Part model, mm, in its own coordinate system. Face numbers are marked on the shaded views. A direction names the side the tool comes from. Coordinates: 2 decimals unless noted, no trailing zeros. Loops run counter-clockwise (first coordinate to the right, second up) from the corner with the lowest first, then second, coordinate; pieces in that order, holes last. Notation, with made-up numbers: M -14.75,68 L -10.75,68 A30 cw -10.75,101 Z; hole C 18.5,-13.5 d5. An arc over 180 degrees is marked long. Use a Markdown table: item, result. Add a question column.
1) Band-saw the part on A-A (z = 10.5). List the corners of the cut face in (x, y).
2) Wall check: probe 1 along X at (y, z) = (-4.5, 17.5); probe 2 along Z at (x, y) = (40, -8.25); probe 3 along X at (y, z) = (-2.25, 3). Give the ranges that are in metal, low to high. Write a range as from..to.
3) Pin check, flat tips, straight feed: pin 1 Ø2 at (x, y) = (33.5, -6.5) entering from +Z; pin 2 Ø1 at (y, z) = (-10, 11.5) entering from -X. Stop position of each tip, or through.
4) Band-saw the part on C-C (z = 18.75). List the corners of the cut face in (x, y), plus the area to 3 significant figures.
5) Pull direction Z, two halves, no side cores. Call the marked faces 3, 4 and 5: released by +Z, released by -Z, zero draft, split by the parting line, or undercut.
6) Tool access for the marked faces 1 and 2: list every direction of +Z, -Z, +X, -X, +Y, -Y with a clear straight run to the whole face (end or side of a thin tool).
7) Band-saw the part on D-D (x = 33.5). List the corners of the cut face in (y, z), plus the area to 3 significant figures.
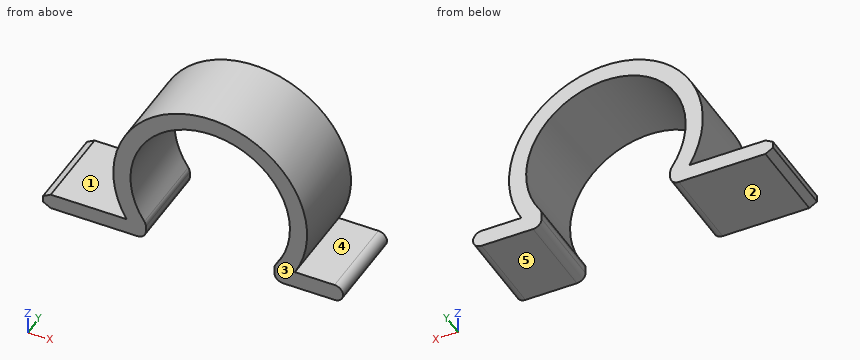
from build123d import *

# Parameters (mm, degrees)
F1_DEPTH   = 12.7
F2_SIZE2   = 0.6599113577
F2_SIZE    = 1.143
F2_2_SIZE2 = 0.6599113577
F2_2_SIZE  = 1.143
F3_R       = 1.26999


# Not quite as in the source:
# - a fillet or chamfer is up to 0.001 mm smaller than in the source, because OpenCascade refuses the exact size


with BuildPart() as f1:
    # F0 (on Front) → F1 (new body)
    with BuildSketch(Plane.XZ):
        with BuildLine():
            Line((0, 2.286), (0, 0))
            Line((0, 0), (15.24, 0))
            Line((15.24, 0), (15.24, 2.54))
            ThreePointArc((15.24, 2.54), (24.765, 21.336682776), (34.29, 2.54))
            Line((34.29, 2.54), (34.29, 0))
            Line((34.29, 0), (44.45, 0))
            Line((44.45, 0), (44.45, 2.54))
            Line((44.45, 2.54), (37.3021676826, 2.54))
            ThreePointArc((37.3021676826, 2.54), (24.6187816105, 23.8759379026), (12.3727573659, 2.286))
            Line((12.3727573659, 2.286), (0, 2.286))
        make_face()
    extrude(amount=F1_DEPTH)

    # F2
    f2_edges = [f1.edges().sort_by_distance(p)[0] for p in [
        (0, -6.35, 0),
    ]]
    f2_side = f1.faces().sort_by_distance((7.62, -6.35, 0))[0]
    chamfer(f2_edges, length=F2_SIZE, length2=F2_SIZE2, reference=f2_side)

    # F2#2
    f2_2_edges = [f1.edges().sort_by_distance(p)[0] for p in [
        (0, -6.35, 2.286),
    ]]
    f2_2_side = f1.faces().sort_by_distance((6.186379, -6.35, 2.286))[0]
    chamfer(f2_2_edges, length=F2_2_SIZE, length2=F2_2_SIZE2, reference=f2_2_side)

    # F3 (radius 1.27 in the source; OpenCascade refuses exactly that, so slightly less here)
    f3_edges = [f1.edges().sort_by_distance(p)[0] for p in [
        (44.45, -6.35, 2.54),
        (44.45, -6.35, 0),
        (34.29, -6.35, 0),
        (34.29, -6.35, 2.54),
        (15.24, -6.35, 2.54),
        (15.24, -6.35, 0),
    ]]
    fillet(f3_edges, radius=F3_R)


solid = f1.part
Entries:
| question | item | result |
|---|---|---|
| 1 | outline | M 10.45,-12.7 L 12.99,-12.7 L 12.99,0 L 10.45,0 Z; M 36.54,-12.7 L 39.08,-12.7 L 39.08,0 L 36.54,0 Z |
| 2 | probe 1 | 12.83..16.05, 33.48..36.7 |
| 2 | probe 2 | 0..2.54 |
| 2 | probe 3 | 11.98..14.92, 34.61..37.55 |
| 3 | pin 1 | z = 21.61 |
| 3 | pin 2 | x = 10.49 |
| 4 | outline | M 13.77,-12.7 L 17.39,-12.7 L 17.39,0 L 13.77,0 Z; M 32.14,-12.7 L 35.76,-12.7 L 35.76,0 L 32.14,0 Z |
| 4 | area | 91.9 mm2 |
| 5 | face 3 | zero draft |
| 5 | face 4 | undercut |
| 5 | face 5 | released by -Z |
| 6 | face 1 | -X, +Y, -Y |
| 6 | face 2 | -Z, +X, -X, +Y, -Y |
| 7 | outline | M -12.7,17.48 L 0,17.48 L 0,20.91 L -12.7,20.91 Z |
| 7 | area | 43.6 mm2 |
